Build history of the part. All positions in model axes, mm. Give positions to 0.01 mm unless a question says otherwise; leave off trailing zeros. Write each loop counter-clockwise with the first axis right and the second up, starting at its lowest first coordinate (ties: lowest second). Pieces come first, ordered by that corner, then holes. Notation, with made-up numbers: M 24,-17 L 66,-17 A21 ccw 66,5 Z; hole C 30,-21.5 d9. An arc over 180 degrees is marked long. Return JSON: item names as keys, results as strings. Group by question number.
Q1. Band-saw the part on A-A, the plane y = -27.5. Give the cut face in (x, z).
Q2. Band-saw the part on C-C, the plane z = 39.5. Give the cut face in (x, y).
Q3. Band-saw the part on D-D, the plane x = 93. Give the cut face in (y, z), then the cut area to 3 significant figures.
Q4. Band-saw the part on B-B, the plane x = 50. Give the cut face in (y, z).
Q5. Wall check: probe 1 along Y at (x, z) = (0, 45.6); probe 2 along Y at (x, z) = (-27.5, 46.5); probe 3 along Z at (x, y) = (-39.5, -69). Give the ranges that are in metal, low to high.
Q6. Flat gauge pins, fed straight in: pin 1 Ø2 at (y, z) = (97.5, 13) entering from -X; pin 2 Ø6 at (x, z) = (-72.5, 28.5) entering from +Y; pin 3 Ø6 at (y, z) = (-25.5, 8) entering from -X. Where does each tip first touch, or does it go through?
from build123d import *

# Parameters (mm, degrees)
SKETCH1_R           = 75
BOSS_EXTRUDE1_DEPTH = 49
SKETCH1_3_R         = 87
SKETCH1_3_R_2       = 75
BOSS_EXTRUDE2_DEPTH = 44.3
SKETCH1_4_R         = 133.5
SKETCH1_4_R_2       = 87
BOSS_EXTRUDE3_DEPTH = 49


with BuildPart() as part:
    # Sketch1 → Boss-Extrude1 (new body)
    with BuildSketch(Plane.XY):
        Circle(SKETCH1_R)
    extrude(amount=BOSS_EXTRUDE1_DEPTH)

    # Sketch1<3> → Boss-Extrude2 (add)
    with BuildSketch(Plane.XY):
        Circle(SKETCH1_3_R)
        Circle(SKETCH1_3_R_2, mode=Mode.SUBTRACT)
    extrude(amount=BOSS_EXTRUDE2_DEPTH)

    # Sketch1<4> → Boss-Extrude3 (add)
    with BuildSketch(Plane.XY):
        Circle(SKETCH1_4_R)
        Circle(SKETCH1_4_R_2, mode=Mode.SUBTRACT)
    extrude(amount=BOSS_EXTRUDE3_DEPTH)


solid = part.part
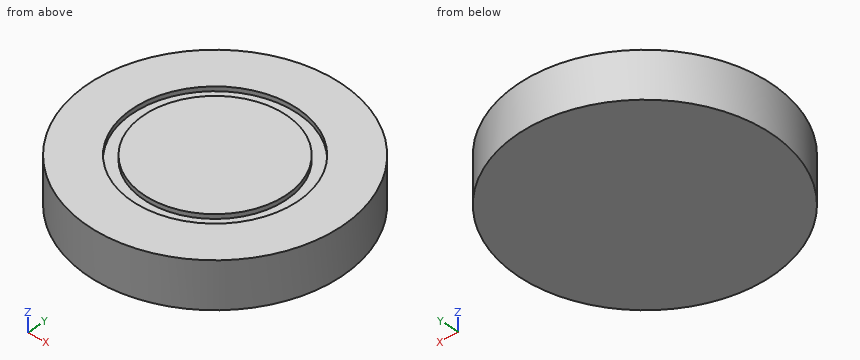
From the geometry:
{
 "1": {"outline": "M -130.64,0 L 130.64,0 L 130.64,49 L 82.54,49 L 82.54,44.3 L 69.78,44.3 L 69.78,49 L -69.78,49 L -69.78,44.3 L -82.54,44.3 L -82.54,49 L -130.64,49 Z"},
 "2": {"outline": "C 0,0 d267"},
 "3": {"outline": "M -95.78,0 L 95.78,0 L 95.78,49 L -95.78,49 Z", "area": "9,390 mm^2"},
 "4": {"outline": "M -123.78,0 L 123.78,0 L 123.78,49 L 71.2,49 L 71.2,44.3 L 55.9,44.3 L 55.9,49 L -55.9,49 L -55.9,44.3 L -71.2,44.3 L -71.2,49 L -123.78,49 Z"},
 "5": {"probe 1": "y = -133.5 to -87, -75 to 75, 87 to 133.5", "probe 2": "y = -130.64 to -82.54, -69.78 to 69.78, 82.54 to 130.64", "probe 3": "z = 0 to 44.3"},
 "6": {"pin 1": "stops at x = -92.25", "pin 2": "stops at y = 113.98", "pin 3": "stops at x = -131.59"}
}
